Print and shaded views of the part. All mm, measured from the part's lowest x, y and z. Round coordinates to 2 decimals unless told otherwise and drop trailing zeros. Write each loop counter-clockwise with the first axis right and the second up, starting at its lowest first coordinate (ties: lowest second). Pieces come first, ordered by that corner, then holes. Notation, with made-up numbers: (64.25, 80) - (92.25, 80) arc R15 ccw to (92.25, 86) - close; hole circle Ø5 at (-28.75, 56.5). An arc over 180 degrees is marked (long way). One line per item, written item: value.
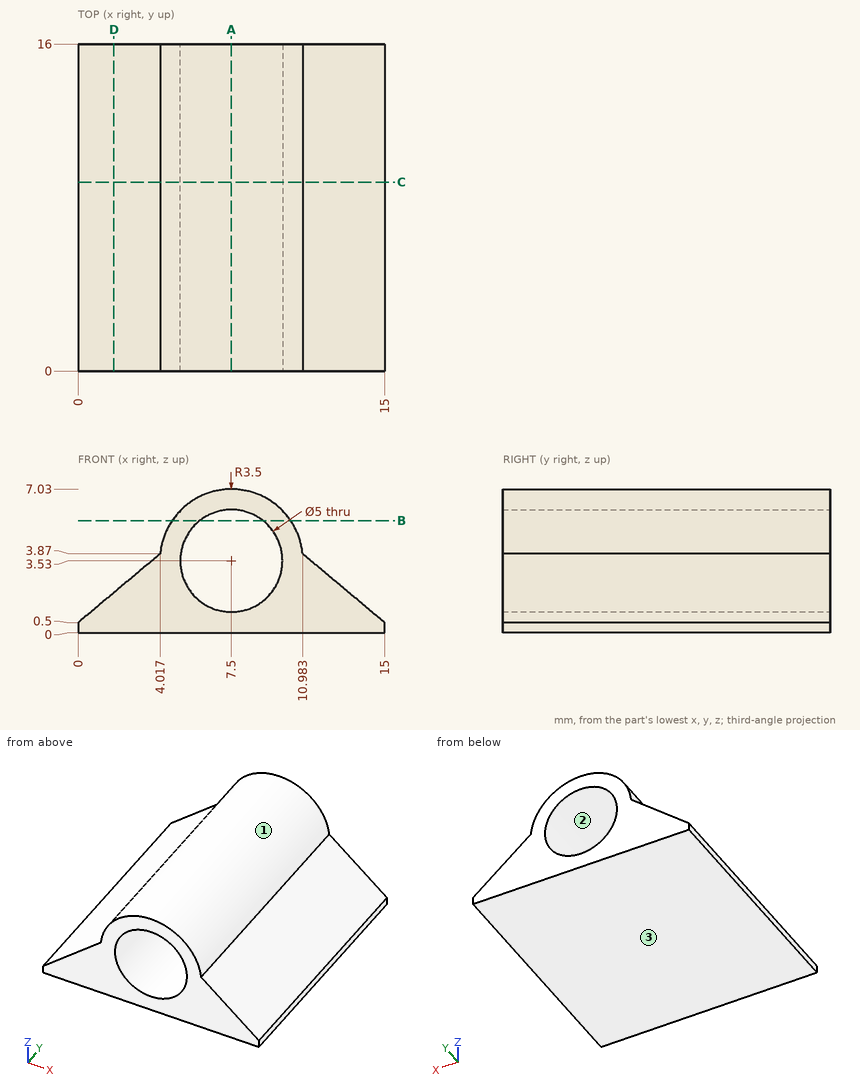
1. Band-saw the part on C-C on y = 9.25. Write the cut outline in (x, z).
Report:
outline: (0, 0) - (15, 0) - (15, 0.5) - (10.98, 3.87) arc R3.5 ccw to (4.02, 3.87) - (0, 0.5) - close; hole circle Ø5 at (7.5, 3.53)
2. Mould opens along X. For the marked faces 1, 2 and 3 say: released by +X, released by -X, zero draft, split by the parting line, or undercut.
Report:
face 1: split by the parting line
face 2: undercut
face 3: zero draft
3. Wall check: probe 1 along Z at (x, y) = (7.5, 6); probe 2 along Z at (x, y) = (5.75, 14.5) (1 decimal); probe 3 along X at (y, z) = (8, 5) (1 decimal). Give the ranges that are in metal, low to high. Write a range as [from, to].
Report:
probe 1: [0, 1.03], [6.03, 7.03]
probe 2: [0, 1.7], [5.3, 6.6]
probe 3: [4.3, 5.5], [9.5, 10.7]
4. Drop flat-ended pins along their axis: pin 1 (2 mm diameter, centred on y = 6.5, z = 4, fed in from +X); pin 2 (5 mm diameter, centred on x = 3, y = 7, fed in from +Z); pin 3 (4 mm diameter, centred on y = 11.5, z = 6, fed in from -X). Give the stop position or say it passes through.
Report:
pin 1: x = 12.02
pin 2: z = 6.4
pin 3: x = 4.03
5. Band-saw the part on B-B on z = 5.5. Write the cut outline in (x, y).
Report:
outline: (4.61, 0) - (5.96, 0) - (5.96, 16) - (4.61, 16) - close; (9.04, 0) - (10.39, 0) - (10.39, 16) - (9.04, 16) - close
6. Band-saw the part on A-A on x = 7.5. Write the cut outline in (y, z).
Report:
outline: (0, 0) - (16, 0) - (16, 1.03) - (0, 1.03) - close; (0, 6.03) - (16, 6.03) - (16, 7.03) - (0, 7.03) - close
7. Band-saw the part on D-D on x = 1.75. Write the cut outline in (y, z), plus the area to 3 significant figures.
Report:
outline: (0, 0) - (16, 0) - (16, 1.97) - (0, 1.97) - close
area: 31.5 mm²
